Geometry: see drawing. Coordinates: mm, zero at the bounding-box minimum. Coordinates: 2 decimals unless noted, no trailing zeros. Loops run counter-clockwise (first coordinate to the right, second up) from the corner with the lowest first, then second, coordinate; pieces in that order, holes last. Notation, with made-up numbers: M 58.5,46.25 L 63.5,46.25 A29 ccw 63.5,66.25 Z; hole C 24.25,41 d7. An arc over 180 degrees is marked long. Write each question's results on one line, items separated by ' | '. Start each with the question number.
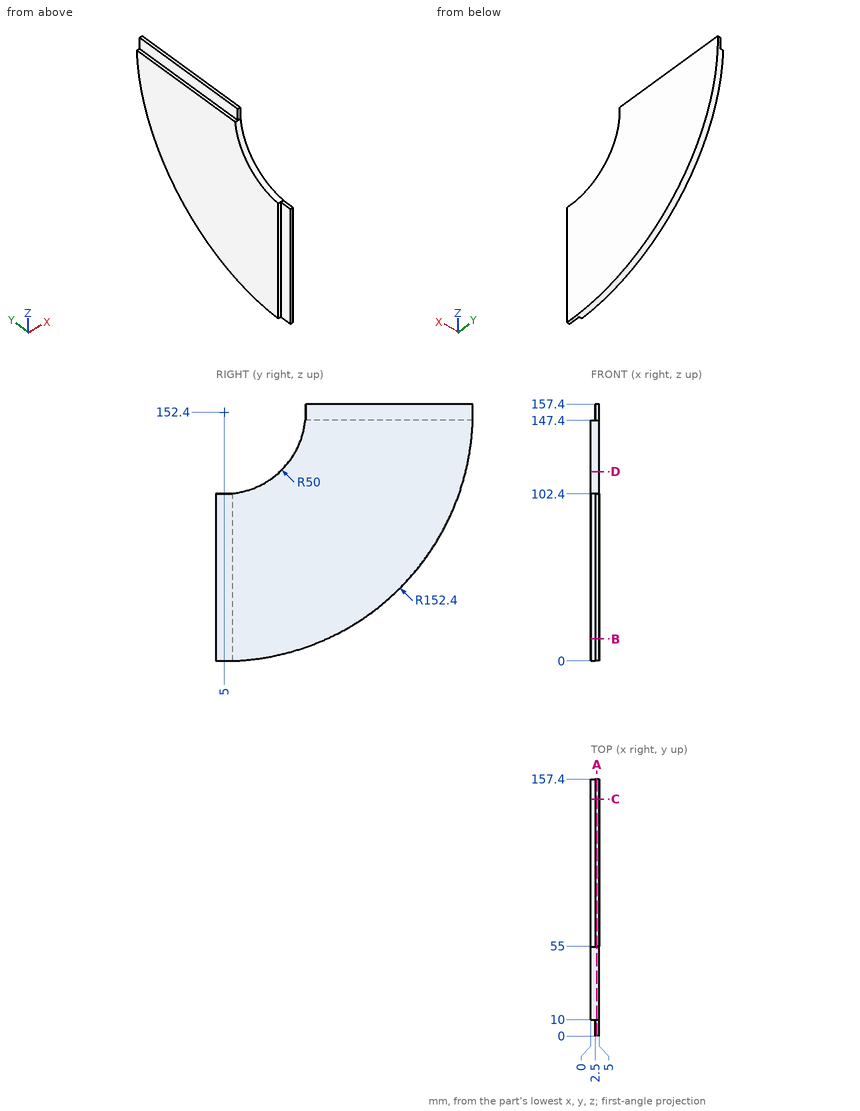
Item 1: Cut plane B-B (z = 13.5). Output: boundary loops of the cut face in (x, y).
Item 2: Cut plane D-D (z = 116). Output: boundary loops of the cut face in (x, y), then the cut area to 3 significant figures.
Item 3: Cut plane C-C (y = 145). Output: boundary loops of the cut face in (x, z).
Item 4: First-contact query: pin 1 Ø8 at (y, z) = (85, 154.5) entering from -X; pin 2 Ø1.2 at (x, y) = (3.5, 3.5) entering from +Z; pin 3 Ø1.2 at (x, z) = (3.5, 150.5) entering from -Y. Flat tips, straight axial feed; report the tip coordinate or a pass-through.
Item 5: Cut plane A-A (x = 3.65). Output: boundary loops of the cut face in (y, z), then the cut area to 3 significant figures.
Item 6: Line query: probe 1 along Z at (x, y) = (3.8, 96); probe 2 along Y at (x, z) = (1.65, 68.5); probe 3 along Y at (x, z) = (0.9, 67). Output: solid intervals per line, ascending.
Response values:
1) outline: M 0,10 L 2.5,10 L 2.5,0 L 5,0 L 5,67.71 L 0,67.71 Z
2) outline: M 0,39.28 L 5,39.28 L 5,152.99 L 0,152.99 Z | area: 569 mm2
3) outline: M 0,92.19 L 5,92.19 L 5,157.4 L 2.5,157.4 L 2.5,147.4 L 0,147.4 Z
4) pin 1: stops at x = 2.5 | pin 2: stops at z = 102.4 | pin 3: stops at y = 55
5) outline: M 0,0.08 A152.4 ccw 157.32,157.4 L 55,157.4 L 55,147.4 L 54.75,147.4 A50 cw 10,102.65 L 10,102.4 L 0,102.4 Z | area: 17,300 mm2
6) probe 1: z = 30.15 to 157.4 | probe 2: y = 10 to 132.23 | probe 3: y = 10 to 131.22
